Work out the finished part from the listing and answer in its coordinate system (mm). Face numbers are marked on the shaded views. A direction names the side the tool comes from. Give positions to 0.01 mm unless a question says otherwise; leave off trailing zeros. Order: outer loops, then holes, each group sorted by start corner. A loop starts at its lowest first (then second) coordinate and runs counter-clockwise, first axis right, second up. Notation, with made-up numbers: (66, 83) - (73, 83) arc R13 ccw to (73, 96) - close; hole circle Ø5 at (59, 13.5). An arc over 180 degrees is marked (long way). Return JSON: item names as keys, results as strings. Group by question number.
from build123d import *

# Parameters (mm, degrees)
F0_R     = 18.6
F0_R_2   = 4.1
F1_DEPTH = 12
F2_R     = 13.5
F2_R_2   = 4.1
F3_DEPTH = 3.7
F5_DEPTH = 4.2


# Not quite as in the source:
# - ends of sketch curves that miss each other by under 0.0002 mm in the source are joined


with BuildPart() as f1:
    # F0 (on Front) → F1 (new body)
    with BuildSketch(Plane.XZ):
        Circle(F0_R)
        Circle(F0_R_2, mode=Mode.SUBTRACT)
    extrude(amount=F1_DEPTH)

    # F2 (on face) → F3 (cut)
    with BuildSketch(Plane.XZ.offset(12)):
        Circle(F2_R)
        Circle(F2_R_2, mode=Mode.SUBTRACT)
    extrude(amount=-F3_DEPTH, mode=Mode.SUBTRACT)

    # F4 (on face) → F5 (cut)
    with BuildSketch(Plane(origin=(0, 0, 0), x_dir=(-1, 0, 0), z_dir=(0, 1, 0))):
        with BuildLine():
            Line((-7.4463871349, 3.4338489537), (-12.3084865507, 6.2402851562))
            ThreePointArc((-12.3084865507, 6.2402851562), (-13.3297808283, 3.5716863063), (-13.7796064717, 0.7499636563))
            Line((-13.7796064717, 0.7499636563), (-8.1665450744, 0.7399605041))
            ThreePointArc((-8.1665450744, 0.7399605041), (-7.9218161925, 2.1177412996), (-7.4463871349, 3.4338489537))
        make_face()
        with BuildLine():
            Line((-0.75, 8.1656291858), (-0.75, 13.7796044936))
            ThreePointArc((-0.75, 13.7796044936), (-3.5717111631, 13.3297741679), (-6.2402985973, 12.3084797362))
            Line((-6.2402985973, 12.3084797362), (-3.4376390894, 7.4446381706))
            ThreePointArc((-3.4376390894, 7.4446381706), (-2.1246263899, 7.9199723928), (-0.75, 8.1656291858))
        make_face()
        with BuildLine():
            ThreePointArc((6.2402985973, 12.3084797362), (3.5717111631, 13.3297741679), (0.75, 13.7796044936))
            Line((0.75, 13.7796044936), (0.75, 8.1656291858))
            ThreePointArc((0.75, 8.1656291858), (2.1246263899, 7.9199723928), (3.4376390894, 7.4446381706))
            Line((3.4376390894, 7.4446381706), (6.2402985973, 12.3084797362))
        make_face()
        with BuildLine():
            Line((7.5393145037, 11.5584919784), (4.7304979814, 6.6979391493))
            ThreePointArc((4.7304979814, 6.6979391493), (5.7956887156, 5.8008613423), (6.6937164195, 4.7364713126))
            Line((6.6937164195, 4.7364713126), (11.5584775515, 7.5393366214))
            ThreePointArc((11.5584775515, 7.5393366214), (9.7580642441, 9.7580829166), (7.5393145037, 11.5584919784))
        make_face()
        with BuildLine():
            Line((12.3084865507, 6.2402851562), (7.4463871349, 3.4338489537))
            ThreePointArc((7.4463871349, 3.4338489537), (7.9218161925, 2.1177412996), (8.1665450744, 0.7399605041))
            Line((8.1665450744, 0.7399605041), (13.7796064717, 0.7499636563))
            ThreePointArc((13.7796064717, 0.7499636563), (13.3297808283, 3.5716863063), (12.3084865507, 6.2402851562))
        make_face()
        with BuildLine():
            ThreePointArc((-6.6937164195, 4.7364713126), (-5.7956887156, 5.8008613423), (-4.7304979814, 6.6979391493))
            Line((-4.7304979814, 6.6979391493), (-7.5393145037, 11.5584919784))
            ThreePointArc((-7.5393145037, 11.5584919784), (-9.7580642441, 9.7580829166), (-11.5584775515, 7.5393366214))
            Line((-11.5584775515, 7.5393366214), (-6.6937164195, 4.7364713126))
        make_face()
        with BuildLine():
            Line((-8.1665450744, -0.7399605041), (-13.7796064717, -0.7499636563))
            ThreePointArc((-13.7796064717, -0.7499636563), (-13.3297808283, -3.5716863063), (-12.3084865507, -6.2402851562))
            Line((-12.3084865507, -6.2402851562), (-7.4463871349, -3.4338489537))
            ThreePointArc((-7.4463871349, -3.4338489537), (-7.9218161925, -2.1177412996), (-8.1665450744, -0.7399605041))
        make_face()
        with BuildLine():
            ThreePointArc((-4.7304979814, -6.6979391493), (-5.7956887156, -5.8008613423), (-6.6937164195, -4.7364713126))
            Line((-6.6937164195, -4.7364713126), (-11.5584775515, -7.5393366214))
            ThreePointArc((-11.5584775515, -7.5393366214), (-9.7580642441, -9.7580829166), (-7.5393145037, -11.5584919784))
            Line((-7.5393145037, -11.5584919784), (-4.7304979814, -6.6979391493))
        make_face()
        with BuildLine():
            ThreePointArc((-0.75, -8.1656291858), (-2.1246263899, -7.9199723928), (-3.4376390894, -7.4446381706))
            Line((-3.4376390894, -7.4446381706), (-6.2402985973, -12.3084797362))
            ThreePointArc((-6.2402985973, -12.3084797362), (-3.5717111631, -13.3297741679), (-0.75, -13.7796044936))
            Line((-0.75, -13.7796044936), (-0.75, -8.1656291858))
        make_face()
        with BuildLine():
            Line((0.75, -8.1656291858), (0.75, -13.7796044936))
            ThreePointArc((0.75, -13.7796044936), (3.5717111631, -13.3297741679), (6.2402985973, -12.3084797362))
            Line((6.2402985973, -12.3084797362), (3.4376390894, -7.4446381706))
            ThreePointArc((3.4376390894, -7.4446381706), (2.1246263899, -7.9199723928), (0.75, -8.1656291858))
        make_face()
        with BuildLine():
            ThreePointArc((6.6937164195, -4.7364713126), (5.7956887156, -5.8008613423), (4.7304979814, -6.6979391493))
            Line((4.7304979814, -6.6979391493), (7.5393145037, -11.5584919784))
            ThreePointArc((7.5393145037, -11.5584919784), (9.7580642441, -9.7580829166), (11.5584775515, -7.5393366214))
            Line((11.5584775515, -7.5393366214), (6.6937164195, -4.7364713126))
        make_face()
        with BuildLine():
            ThreePointArc((8.1665450744, -0.7399605041), (7.9218161925, -2.1177412996), (7.4463871349, -3.4338489537))
            Line((7.4463871349, -3.4338489537), (12.3084865507, -6.2402851562))
            ThreePointArc((12.3084865507, -6.2402851562), (13.3297761181, -3.5717038849), (13.7796044936, -0.75))
            Line((13.7796044936, -0.75), (8.1665450744, -0.7399605041))
        make_face()
    extrude(amount=-F5_DEPTH, mode=Mode.SUBTRACT)

    # F6 (on Right) → F7 (revolve, cut)
    with BuildSketch(Plane.YZ):
        with BuildLine():
            ThreePointArc((-12.0048904791, 18.2), (-6.0048904791, 18.6146934366), (-0.0048904791, 18.2))
            Line((-0.0048904791, 18.2), (0.3708341392, 18.1622945595))
            Line((0.3708341392, 18.1622945595), (0.3708341392, 18.6))
            Line((0.3708341392, 18.6), (0.3567633394, 19.1855213957))
            Line((0.3567633394, 19.1855213957), (-12.2980514625, 19.1855213957))
            Line((-12.2980514625, 19.1855213957), (-12.27635841, 18.5901094228))
            Line((-12.27635841, 18.5901094228), (-12.27635841, 18.1622945595))
            Line((-12.27635841, 18.1622945595), (-12.0048904791, 18.2))
        make_face()
    revolve(axis=Axis((0, -2.5395685887, 0), (0, 1, 0)), mode=Mode.SUBTRACT)


solid = f1.part
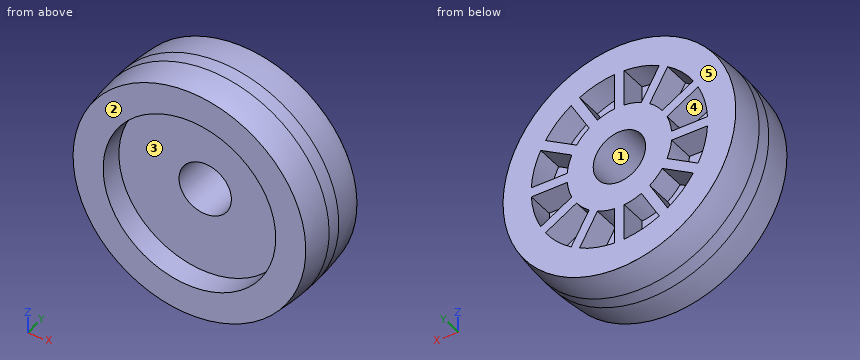
1. Consider probe 1 along Z at (x, y) = (0, -4.75); probe 2 along X at (y, z) = (-3, 12.5); probe 3 along Y at (x, z) = (1, 9.5). Determine where each line is inside the solid, lowest interval first. Write a range as from..to.
2. The part is cut by section A-A (y = -6.5). Give the vertices of the cut face in (x, z), and give its area (3 significant figures).
3. Each of these flat-tipped pins is pushed along its axis until it touches: pin 1 (5.5 mm diameter, centred on x = -8.5, z = 10, fed in from +Y); pin 2 (1 mm diameter, centred on x = 3, y = -8, fed in from -Z); pin 3 (3 mm diameter, centred on x = -11, y = -10, fed in from +Z); pin 4 (1.6 mm diameter, centred on x = 2, z = 12, fed in from +Y). Where does it stop, or does it pass through?
4. Determine the mould class of the marked faces 1 and 2 for opening direction Z: released by +Z, released by -Z, zero draft, split by the parting line, or undercut.
5. A tool of negligible diameter and unlimited length cuts with its end or side. For the marked faces 3, 4 and 5, from which of +Z, -Z, +X, -X, +Y, -Y can it reach the whole face along a straight path? Write none if from no direction.
6. The part is cut by section B-B (y = -2.25). State how many separate pieces and enclosed holes the cut face has, and give its area (3 significant figures).
Answers:
{
 "1": {"probe 1": "z = -18.6..-4.1, 4.1..18.6", "probe 2": "x = -13.65..-5.85, -0.75..0.75, 5.85..13.65", "probe 3": "y = -8.3..-4.2"},
 "2": {"outline": "circle Ø37.2 at (0, 0); hole circle Ø8.2 at (0, 0)", "area": "1,030 mm^2"},
 "3": {"pin 1": "stops at y = 0", "pin 2": "stops at z = -18.4", "pin 3": "stops at z = 15.81", "pin 4": "stops at y = -4.2"},
 "4": {"face 1": "undercut", "face 2": "zero draft"},
 "5": {"face 3": "-Y", "face 4": "+Y", "face 5": "+Z, -Z, +X, -X, +Y"},
 "6": {"separate pieces": "1", "enclosed holes": "13", "area": "731 mm^2"}
}
